from build123d import *

# Parameters (mm, degrees)
BOSS_EXTRUDE1_DEPTH = 9.75
CUT_EXTRUDE3_START  = -4.875
CUT_EXTRUDE3_DEPTH  = 4.875


with BuildPart() as part:
    # Sketch1 → Boss-Extrude1 (new body)
    with BuildSketch(Plane(origin=(0, 0, 0), x_dir=(1, 0, 0), z_dir=(0, 1, 0))):
        with BuildLine():
            Line((0, 5), (0, 0))
            Line((0, 0), (43.45, 0))
            ThreePointArc((43.45, 0), (44.914466094, 3.535533906), (48.45, 5))
            Line((48.45, 5), (0, 5))
        make_face()
        with BuildLine():
            Line((43.45, 0), (0, 0))
            Line((0, 0), (0, -5.049027621))
            Line((0, -5.049027621), (48.45, -5.049027621))
            Line((48.45, -5.049027621), (48.45, -5))
            ThreePointArc((48.45, -5), (44.914466094, -3.535533906), (43.45, 0))
        make_face()
        with BuildLine():
            ThreePointArc((53.45, 0), (51.985533906, 3.535533906), (48.45, 5))
            Line((48.45, 5), (48.45, 1.5))
            ThreePointArc((48.45, 1.5), (49.510660172, 1.060660172), (49.95, 0))
            ThreePointArc((49.95, 0), (49.510660172, -1.060660172), (48.45, -1.5))
            Line((48.45, -1.5), (48.45, -5))
            ThreePointArc((48.45, -5), (51.985533906, -3.535533906), (53.45, 0))
        make_face()
        with BuildLine():
            ThreePointArc((48.45, 5), (44.914466094, 3.535533906), (43.45, 0))
            Line((43.45, 0), (46.95, 0))
            ThreePointArc((46.95, 0), (47.389339828, 1.060660172), (48.45, 1.5))
            Line((48.45, 1.5), (48.45, 5))
        make_face()
        with BuildLine():
            Line((46.95, 0), (43.45, 0))
            ThreePointArc((43.45, 0), (44.914466094, -3.535533906), (48.45, -5))
            Line((48.45, -5), (48.45, -1.5))
            ThreePointArc((48.45, -1.5), (47.389339828, -1.060660172), (46.95, 0))
        make_face()
    boss_extrude1 = extrude(amount=BOSS_EXTRUDE1_DEPTH)

    # Mirror1: Boss-Extrude1 across plane
    add(boss_extrude1.mirror(Plane(origin=(0, 0, 0), x_dir=(0, 0, 1), z_dir=(1, 0, 0))))

    # Sketch2 → Cut-Extrude3 (cut)
    with BuildSketch(Plane(origin=(0, 9.75, 0), x_dir=(1, 0, 0), z_dir=(0, 1, 0)).offset(CUT_EXTRUDE3_START)):
        with BuildLine():
            Line((49.95, 0), (53.45, 0))
            ThreePointArc((53.45, 0), (51.985533906, 3.535533906), (48.45, 5))
            Line((48.45, 5), (43.45, 5))
            Line((43.45, 5), (43.45, 0))
            Line((43.45, 0), (46.95, 0))
            ThreePointArc((46.95, 0), (48.45, 1.5), (49.95, 0))
        make_face()
        with BuildLine():
            ThreePointArc((48.45, -5), (51.985533906, -3.535533906), (53.45, 0))
            Line((53.45, 0), (49.95, 0))
            ThreePointArc((49.95, 0), (48.45, -1.5), (46.95, 0))
            Line((46.95, 0), (43.45, 0))
            Line((43.45, 0), (43.45, -5.049027621))
            Line((43.45, -5.049027621), (48.45, -5.049027621))
            Line((48.45, -5.049027621), (48.45, -5))
        make_face()
    cut_extrude3 = extrude(amount=CUT_EXTRUDE3_DEPTH, mode=Mode.SUBTRACT)

    # Mirror2: Cut-Extrude3 across plane
    add(cut_extrude3.mirror(Plane(origin=(0, 0, 0), x_dir=(0, 0, 1), z_dir=(1, 0, 0))), mode=Mode.SUBTRACT)


solid = part.part
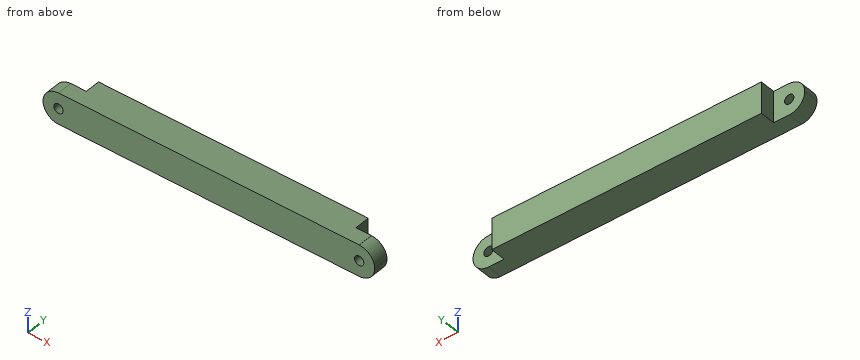
Part model, mm, in its own coordinate system. Coordinates: 2 decimals unless noted, no trailing zeros. Loops run counter-clockwise (first coordinate to the right, second up) from the corner with the lowest first, then second, coordinate; pieces in that order, holes last. Notation, with made-up numbers: M 49.5,36.25 L 81.5,36.25 A8 ccw 81.5,44.25 Z; hole C -17,42.5 d6. An arc over 180 degrees is marked long. Use a Markdown table: item, result. Add a question column.
Q1. Probe L1, parallel to X at y = 1, z = -0.25; L2, parallel to X at y = 1.25, z = 1; L3, parallel to X at y = 5.5, z = -4.5. List the from-to ranges inside material, lowest first.
Q2. Cut at A-A (y = 1). Write the cut outline in (x, z).
Q3. Cut at B-B (z = -4). Write the cut outline in (x, y) (3 decimals), and give its area (3 significant figures).
Q4. Pin check, flat tips, straight feed: P1, Ø3, axis at x = 49.5, z = 0.5, coming from the +Y side (3 decimals); P2, Ø1.5, axis at y = 7.5, z = -1.5, coming from the -X side; P3, Ø1, axis at y = 4, z = 2.5, coming from the +X side. Stop position of each tip, or through.
Q5. Cut at C-C (z = 3). Write the cut outline in (x, y) (3 decimals), and give its area (3 significant figures).
Q6. Cut at D-D (y = 6.75). Write the cut outline in (x, z).
Worked out:
| question | item | result |
|---|---|---|
| 1 | L1 | x = -53.44 to -49.93, -46.97 to 46.97, 49.93 to 53.44 |
| 1 | L2 | x = -53.35 to -49.57, -47.33 to 47.33, 49.57 to 53.35 |
| 1 | L3 | x = -43.45 to 43.45 |
| 2 | outline | M -48.45,-5 L 48.45,-5 A5 ccw 48.45,5 L 48.45,5.05 L -48.45,5.05 L -48.45,5 A5 ccw Z; hole C -48.45,0 d3; hole C 48.45,0 d3 |
| 3 | outline | M -51.45,0 L 51.45,0 L 51.45,4.875 L 43.45,4.875 L 43.45,9.75 L -43.45,9.75 L -43.45,4.875 L -51.45,4.875 Z |
| 3 | area | 925 mm2 |
| 4 | P1 | stops at y = 4.875 |
| 4 | P2 | stops at x = -43.45 |
| 4 | P3 | stops at x = 53.03 |
| 5 | outline | M -52.45,0 L 52.45,0 L 52.45,4.875 L 43.45,4.875 L 43.45,9.75 L -43.45,9.75 L -43.45,4.875 L -52.45,4.875 Z |
| 5 | area | 935 mm2 |
| 6 | outline | M -43.45,-5 L 43.45,-5 L 43.45,5.05 L -43.45,5.05 Z |
